Verification items for the finished model (mm, model axes). A direction names the side the tool comes from. Round coordinates to 2 decimals unless told otherwise and drop trailing zeros. Loops run counter-clockwise (first coordinate to the right, second up) from the corner with the lowest first, then second, coordinate; pieces in that order, holes last. Notation, with made-up numbers: (-0.75, -31) -> (6.25, -31) arc R19 ccw to (6.25, -5) -> close; hole circle Ø3 at (40.25, 37). An arc over 180 degrees is marked (long way). Write item = value, one per line. Start each with the question number.
```python
from build123d import *

# Parameters (mm, degrees)
BOSS_EXTRUDE1_DEPTH     = 6.3
CHAMFER3_SIZE           = 2
CUT_EXTRUDE2_DEPTH      = 0.79
SKETCH6_W               = 0.775
SKETCH6_H               = 6.713276343
CUT_EXTRUDE4_DEPTH      = 0.79
CUT_EXTRUDE6_DEPTH      = 1.79
CUT_EXTRUDE6_DEPTH_BACK = 6.21


with BuildPart() as part:
    # Sketch1 → Boss-Extrude1 (new body)
    with BuildSketch(Plane(origin=(0, 0, 0), x_dir=(0, 0, -1), z_dir=(1, 0, 0))):
        with BuildLine():
            Line((0, 0.1), (0, 7.11))
            Line((0, 7.11), (-0.241393443, 8.21))
            Line((-0.241393443, 8.21), (-0.647131148, 8.21))
            Line((-0.647131148, 8.21), (-0.79, 7.11))
            Line((-0.79, 7.11), (-0.79, -0.04))
            ThreePointArc((-0.79, -0.04), (-0.570330086, -0.570330086), (-0.04, -0.79))
            Line((-0.04, -0.79), (5.21, -0.79))
            Line((5.21, -0.79), (5.21, 0))
            Line((5.21, 0), (0.1, 0))
            ThreePointArc((0.1, 0), (0.029289322, 0.029289322), (0, 0.1))
        make_face()
    extrude(amount=BOSS_EXTRUDE1_DEPTH)

    # Chamfer3
    chamfer3_edges = [part.edges().sort_by_distance(p)[0] for p in [
        (0, -0.395, -5.21),
        (6.3, -0.395, -5.21),
    ]]
    chamfer(chamfer3_edges, length=CHAMFER3_SIZE)

    # Sketch5 → Cut-Extrude2 (cut)
    with BuildSketch(Plane.XY.offset(0.79)):
        with BuildLine():
            Line((2.730622244, 5.808829869), (2.026555611, 3.890729922))
            ThreePointArc((2.026555611, 3.890729922), (3.20000017, 2.21), (4.373444272, 3.890730241))
            Line((4.373444272, 3.890730241), (3.669633952, 5.808130298))
            ThreePointArc((3.669633952, 5.808130298), (3.200372504, 6.136537762), (2.730622244, 5.808829869))
        make_face()
    extrude(amount=-CUT_EXTRUDE2_DEPTH, mode=Mode.SUBTRACT)

    # Sketch6 → Cut-Extrude4 (cut)
    with BuildSketch(Plane(origin=(0, 0, 0), x_dir=(-1, 0, 0), z_dir=(0, 0, -1))):
        with Locations((-5.9125, 4.853361829)):
            Rectangle(SKETCH6_W, SKETCH6_H)
        with Locations((-0.3875, 4.853361829)):
            Rectangle(SKETCH6_W, SKETCH6_H)
    extrude(amount=-CUT_EXTRUDE4_DEPTH, mode=Mode.SUBTRACT)

    # Sketch4 → Cut-Extrude6 (cut, two sides)
    with BuildSketch(Plane.XY) as cut_extrude6_sk:
        Polygon((2.275, 8.21), (0.775, 8.21), (0.755504439, 6.71), align=None)
        Polygon((5.544495561, 6.71), (4.025, 8.21), (5.525, 8.21), align=None)
    extrude(amount=CUT_EXTRUDE6_DEPTH, mode=Mode.SUBTRACT)
    extrude(cut_extrude6_sk.sketch, amount=-CUT_EXTRUDE6_DEPTH_BACK, mode=Mode.SUBTRACT)


solid = part.part
```
(1) Section check C-C on z = -0.75. Enter the section's corners in (x, y).
(2) Section check A-A on x = 3.2. Enter the section's corners in (y, z), then the cut area to 3 significant figures.
(3) Draft check along Y on faces 1 (the flat face through (4.786, 7.459, 0.389)), 2 (the cylindrical face through (3.17, 2.21, 0.4)), 3 (the flat face through (0, -0.4, -0.7)). Enter one of: +Y half, -Y half, draft (parallel to the pull), parting line (faces both ways), or undercut.
(4) Section check B-B on y = 3.46. Enter the section's corners in (x, z) (3 decimals), then the cut area to 3 significant figures.
(5) Section check D-D on y = 2.5. Enter the section's corners in (x, z) (3 decimals), then the cut area to 3 significant figures.
(6) Access from +Z, -Z, +X, -X, +Y, -Y to the whole of each face (thin tool, end or side, straight path). Record for faces 4 (the flat face through (3, -0.79, -3)), 5 (the flat face through (3, 2, 0)).
(7) Scan lines: line 1 (X direction, y = 3.46, z = 0.4) (3 decimals); line 2 (Y direction, x = 1, z = -1); line 3 (Y direction, x = 3.2, z = 0.4). Record each from-to range of solid material in increasing order. Write a range as [from, to].
(8) Depth check by flat-ended pin: pin 1 Ø0.6 at (x, z) = (6, 0.5) entering from +Y; pin 2 Ø1.9 at (x, y) = (2.5, 5) entering from -Z; pin 3 Ø2 at (x, y) = (3.2, 3.46) entering from -Z; pin 4 Ø1.5 at (x, z) = (4.5, -3) entering from +Y. Enter the tip coordinate at first touch or a pass-through.
Computed values:
q1.outline = (0, -0.79) -> (6.3, -0.79) -> (6.3, 0) -> (0, 0) -> close
q2.outline = (-0.79, -5.21) -> (0, -5.21) -> (0, -0.1) arc R0.1 cw to (0.1, 0) -> (2.21, 0) -> (2.21, 0.79) -> (-0.04, 0.79) arc R0.75 ccw to (-0.79, 0.04) -> close; (6.14, 0) -> (7.11, 0) -> (8.21, 0.24) -> (8.21, 0.65) -> (7.11, 0.79) -> (6.14, 0.79) -> close
q2.area = 7.79 mm²
q3.face_1 = +Y half
q3.face_2 = undercut
q3.face_3 = draft
q4.outline = (0.775, 0) -> (1.95, 0) -> (1.95, 0.79) -> (0.775, 0.79) -> close; (4.45, 0) -> (5.525, 0) -> (5.525, 0.79) -> (4.45, 0.79) -> close
q4.area = 1.78 mm²
q5.outline = (0.775, 0) -> (2.399, 0) -> (2.399, 0.79) -> (0.775, 0.79) -> close; (4.001, 0) -> (5.525, 0) -> (5.525, 0.79) -> (4.001, 0.79) -> close
q5.area = 2.49 mm²
q6.face_4 = +Z, -Z, +X, -X, -Y
q6.face_5 = -Z, +X, -X, +Y
q7.line_1 = [0.775, 1.95], [4.45, 5.525]
q7.line_2 = [-0.79, 0]
q7.line_3 = [-0.7, 2.21], [6.14, 8.21]
q8.pin_1 = 1.5
q8.pin_2 = 0
q8.pin_3 = through
q8.pin_4 = 0
